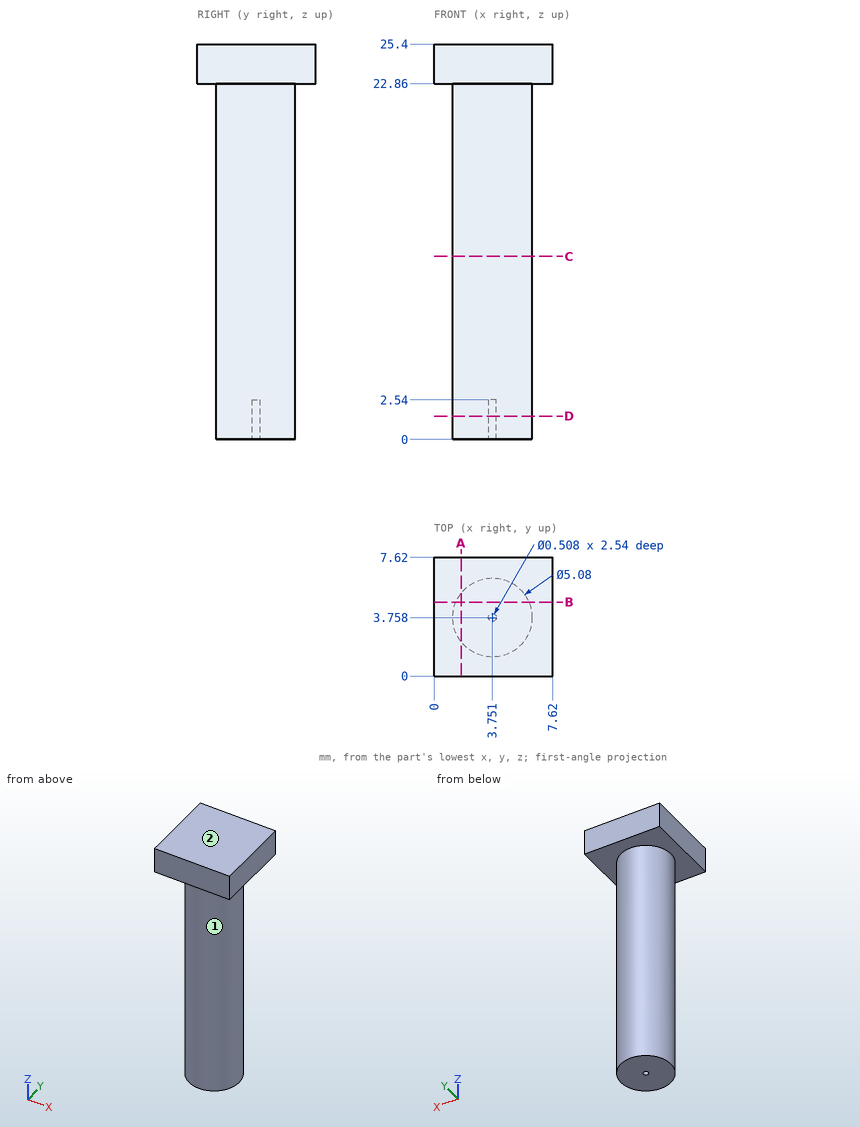
Print and shaded views of the part. All mm, measured from the part's lowest x, y and z. A direction names the side the tool comes from. Round coordinates to 2 decimals unless told otherwise and drop trailing zeros. Order: outer loops, then holes, each group sorted by start corner. A loop starts at its lowest first (then second) coordinate and runs counter-clockwise, first axis right, second up.
Q1. Drop flat-ended pins along their axis: pin 1 (1 mm diameter, centred on y = 5.5, z = 3, fed in from +X); pin 2 (4 mm diameter, centred on x = 4.5, z = 8, fed in from -Y). Give the stop position or say it passes through.
Q2. Slice it at A-A (x = 1.75). Write the cut outline in (y, z).
Q3. Slice it at B-B (y = 4.75). Write the cut outline in (x, z).
Q4. Slice it at D-D (z = 1.5). Write the cut outline in (x, y) (1 decimal), and give its area (3 significant figures).
Q5. Which spindle directions (+Z, -Z, +X, -X, +Y, -Y) get a long thin tool onto all of the face, cutting with end or side? Do the marked faces 1 and 2. Say none if no direction does.
Q6. Slice it at C-C (z = 11.75). Write the cut outline in (x, y), and give its area (3 significant figures).
Q7. Wall check: L1, parallel to Z at x = 6.5, y = 3.5; L2, parallel to Y at x = 3.75, z = 16.75; L3, parallel to X at y = 3.75, z = 10.25. Give the ranges that are in metal, low to high.
Results below:
1. pin 1: stops at x = 5.97
1. pin 2: stops at y = 1.22
2. outline: (0, 22.86) - (2.19, 22.86) - (2.19, 0) - (5.32, 0) - (5.32, 22.86) - (7.62, 22.86) - (7.62, 25.4) - (0, 25.4) - close
3. outline: (0, 22.86) - (1.41, 22.86) - (1.41, 0) - (6.09, 0) - (6.09, 22.86) - (7.62, 22.86) - (7.62, 25.4) - (0, 25.4) - close
4. outline: circle Ø5.1 at (3.8, 3.8); hole circle Ø0.5 at (3.8, 3.8)
4. area: 20.1 mm2
5. face 1: -Z
5. face 2: +Z, +X, -X, +Y, -Y
6. outline: circle Ø5.08 at (3.75, 3.76)
6. area: 20.3 mm2
7. L1: z = 22.86 to 25.4
7. L2: y = 1.22 to 6.3
7. L3: x = 1.21 to 6.29
